```python
from build123d import *

# Parameters (mm, degrees)
CROQUIS1_W              = 45
CROQUIS1_H              = 45
SALIENTE_EXTRUIR1_DEPTH = 10
CORTAR_EXTRUIR1_DEPTH   = 10
CROQUIS3_W              = 26
CROQUIS3_H              = 26
CORTAR_EXTRUIR5_DEPTH   = 8
CROQUIS4_W              = 12
CROQUIS4_H              = 11
CORTAR_EXTRUIR6_DEPTH   = 4
CORTAR_EXTRUIR7_DEPTH   = 4
CROQUIS6_R              = 1.5
CORTAR_EXTRUIR8_DEPTH   = 24
CROQUIS7_R              = 1.5
CORTAR_EXTRUIR9_DEPTH   = 8


with BuildPart() as part:
    # Croquis1 → Saliente-Extruir1 (new body)
    with BuildSketch(Plane.XY):
        Rectangle(CROQUIS1_W, CROQUIS1_H)
    extrude(amount=SALIENTE_EXTRUIR1_DEPTH)

    # Croquis2 → Cortar-Extruir1 (cut)
    with BuildSketch(Plane.XY.offset(10)):
        with BuildLine():
            ThreePointArc((-11.5, -6), (-7.610912703, -7.610912703), (-6, -11.5))
            Line((-6, -11.5), (6, -11.5))
            ThreePointArc((6, -11.5), (7.610912703, -7.610912703), (11.5, -6))
            Line((11.5, -6), (11.5, 6))
            ThreePointArc((11.5, 6), (7.610912703, 7.610912703), (6, 11.5))
            Line((6, 11.5), (-6, 11.5))
            ThreePointArc((-6, 11.5), (-7.610912703, 7.610912703), (-11.5, 6))
            Line((-11.5, 6), (-11.5, -6))
        make_face()
    extrude(amount=-CORTAR_EXTRUIR1_DEPTH, mode=Mode.SUBTRACT)

    # Croquis3 → Cortar-Extruir5 (cut)
    with BuildSketch(Plane.XY.offset(10)):
        Rectangle(CROQUIS3_W, CROQUIS3_H)
    extrude(amount=-CORTAR_EXTRUIR5_DEPTH, mode=Mode.SUBTRACT)

    # Croquis4 → Cortar-Extruir6 (cut)
    with BuildSketch(Plane(origin=(0, 0, 0), x_dir=(-1, 0, 0), z_dir=(0, 0, -1))):
        with Locations((0, 17)):
            Rectangle(CROQUIS4_W, CROQUIS4_H)
    extrude(amount=-CORTAR_EXTRUIR6_DEPTH, mode=Mode.SUBTRACT)

    # Croquis5 → Cortar-Extruir7 (cut)
    with BuildSketch(Plane(origin=(0, 0, 0), x_dir=(-1, 0, 0), z_dir=(0, 0, -1))):
        with BuildLine():
            ThreePointArc((-7.6, 9), (-9.989949494, 9.989949494), (-9, 7.6))
            Line((-9, 7.6), (-9, 9))
            Line((-9, 9), (-7.6, 9))
        make_face()
        with BuildLine():
            Line((-9, 9), (-9, 7.6))
            ThreePointArc((-9, 7.6), (-8.010050506, 8.010050506), (-7.6, 9))
            Line((-7.6, 9), (-9, 9))
        make_face()
        with BuildLine():
            ThreePointArc((7.6, 9), (8.010050506, 8.010050506), (9, 7.6))
            Line((9, 7.6), (9, 9))
            Line((9, 9), (7.6, 9))
        make_face()
        with BuildLine():
            Line((9, 9), (9, 7.6))
            ThreePointArc((9, 7.6), (9.989949494, 8.010050506), (10.4, 9))
            ThreePointArc((10.4, 9), (9, 10.4), (7.6, 9))
            Line((7.6, 9), (9, 9))
        make_face()
        with BuildLine():
            ThreePointArc((9, -7.6), (8.010050506, -8.010050506), (7.6, -9))
            Line((7.6, -9), (9, -9))
            Line((9, -9), (9, -7.6))
        make_face()
        with BuildLine():
            Line((9, -9), (7.6, -9))
            ThreePointArc((7.6, -9), (9, -10.4), (10.4, -9))
            ThreePointArc((10.4, -9), (9.989949494, -8.010050506), (9, -7.6))
            Line((9, -7.6), (9, -9))
        make_face()
        with BuildLine():
            Line((-9, -7.6), (-9, -9))
            Line((-9, -9), (-7.6, -9))
            ThreePointArc((-7.6, -9), (-8.010050506, -8.010050506), (-9, -7.6))
        make_face()
        with BuildLine():
            Line((-7.6, -9), (-9, -9))
            Line((-9, -9), (-9, -7.6))
            ThreePointArc((-9, -7.6), (-9.989949494, -9.989949494), (-7.6, -9))
        make_face()
    extrude(amount=-CORTAR_EXTRUIR7_DEPTH, mode=Mode.SUBTRACT)

    # Croquis6 → Cortar-Extruir8 (cut)
    with BuildSketch(Plane(origin=(0, 0, 0), x_dir=(-1, 0, 0), z_dir=(0, 0, -1))):
        with Locations((-17.5, 17.5)):
            Circle(CROQUIS6_R)
        with Locations((-17.5, -17.5)):
            Circle(CROQUIS6_R)
        with Locations((17.5, -17.5)):
            Circle(CROQUIS6_R)
        with Locations((17.5, 17.5)):
            Circle(CROQUIS6_R)
    extrude(amount=-CORTAR_EXTRUIR8_DEPTH, mode=Mode.SUBTRACT)

    # Croquis7 → Cortar-Extruir9 (cut)
    # profile 1 of 4: a face of its own
    with BuildSketch(Plane(origin=(0, 0, 0), x_dir=(-1, 0, 0), z_dir=(0, 0, -1))):
        with BuildLine():
            Line((-22.5, 22.5), (-22.5, 10.5))
            ThreePointArc((-22.5, 10.5), (-14.014718626, 14.014718626), (-10.5, 22.5))
            Line((-10.5, 22.5), (-22.5, 22.5))
        make_face()
        with Locations((-17.5, 17.5)):
            Circle(CROQUIS7_R, mode=Mode.SUBTRACT)
    # profile 2 of 4: a face of its own
    with BuildSketch(Plane(origin=(0, 0, 0), x_dir=(-1, 0, 0), z_dir=(0, 0, -1))):
        with BuildLine():
            ThreePointArc((10.5, 22.5), (14.014718626, 14.014718626), (22.5, 10.5))
            Line((22.5, 10.5), (22.5, 22.5))
            Line((22.5, 22.5), (10.5, 22.5))
        make_face()
        with Locations((17.5, 17.5)):
            Circle(CROQUIS7_R, mode=Mode.SUBTRACT)
    # profile 3 of 4: a face of its own
    with BuildSketch(Plane(origin=(0, 0, 0), x_dir=(-1, 0, 0), z_dir=(0, 0, -1))):
        with BuildLine():
            Line((10.5, -22.5), (22.5, -22.5))
            Line((22.5, -22.5), (22.5, -10.5))
            ThreePointArc((22.5, -10.5), (14.014718626, -14.014718626), (10.5, -22.5))
        make_face()
        with Locations((17.5, -17.5)):
            Circle(CROQUIS7_R, mode=Mode.SUBTRACT)
    # profile 4 of 4: a face of its own
    with BuildSketch(Plane(origin=(0, 0, 0), x_dir=(-1, 0, 0), z_dir=(0, 0, -1))):
        with BuildLine():
            Line((-22.5, -22.5), (-10.5, -22.5))
            ThreePointArc((-10.5, -22.5), (-14.014718626, -14.014718626), (-22.5, -10.5))
            Line((-22.5, -10.5), (-22.5, -22.5))
        make_face()
        with Locations((-17.5, -17.5)):
            Circle(CROQUIS7_R, mode=Mode.SUBTRACT)
    extrude(amount=-CORTAR_EXTRUIR9_DEPTH, mode=Mode.SUBTRACT)


solid = part.part
```
Geometry: final body of the model. Coordinates: model frame, mm. A direction names the side the tool comes from. Coordinates: 2 decimals unless noted, no trailing zeros. Order: outer loops, then holes, each group sorted by start corner. A loop starts at its lowest first (then second) coordinate and runs counter-clockwise, first axis right, second up. Notation, with made-up numbers: (87, 52) - (94, 52) arc R29 cw to (94, 79) - close; hole circle Ø3 at (-6, 39). An arc over 180 degrees is marked (long way). Write each question's results on one line, items separated by ' | '.
1) Section C-C, the plane y = 17.5. Return loops of the section in (x, z), plus the area to 3 significant figures.
Results list:
outline: (-22.5, 8) - (-19, 8) - (-19, 10) - (-22.5, 10) - close; (-16, 8) - (-11.59, 8) - (-11.59, 0) - (-6, 0) - (-6, 4) - (6, 4) - (6, 0) - (11.59, 0) - (11.59, 8) - (16, 8) - (16, 10) - (-16, 10) - close; (19, 8) - (22.5, 8) - (22.5, 10) - (19, 10) - close | area: 215 mm^2
2) Pin query (flat end, axial travel): pin 1 (13 mm diameter, centred on x = -15, y = -18, fed in from -Z); pin 2 (3 mm diameter, centred on y = 19, z = 1, fed in from -X); pin 3 (3 mm diameter, centred on x = -17.5, z = 1, fed in from -Y); pin 4 (3 mm diameter, centred on x = -13, z = 3.5, fed in from -Y). Return the tip coordinate at first contact, or that it passes through.
Results list:
pin 1: z = 0 | pin 2: x = -11.59 | pin 3: y = -12.41 | pin 4: y = -17.7
3) Line query: line 1 (Y direction, x = 17.5, z = 9); line 2 (Y direction, x = 9, z = 1.1); line 3 (X direction, y = 6, z = 7.5). Output: solid intervals per line, ascending. Write a range as from..to.
Results list:
line 1: -22.5..-19, -16..16, 19..22.5 | line 2: -22.5..-10.4, -7.6..-6.6, 6.6..7.6, 10.4..22.5 | line 3: -22.5..-13, 13..22.5
4) Section D-D, the plane x = 17.5. Return loops of the section in (y, z).
Results list:
outline: (-22.5, 8) - (-19, 8) - (-19, 10) - (-22.5, 10) - close; (-16, 8) - (-11.59, 8) - (-11.59, 0) - (11.59, 0) - (11.59, 8) - (16, 8) - (16, 10) - (-16, 10) - close; (19, 8) - (22.5, 8) - (22.5, 10) - (19, 10) - close
5) Section A-A, the plane x = 3. Return loops of the section in (y, z), plus the area to 3 significant figures.
Results list:
outline: (-22.5, 0) - (-11.5, 0) - (-11.5, 2) - (-13, 2) - (-13, 10) - (-22.5, 10) - close; (13, 4) - (22.5, 4) - (22.5, 10) - (13, 10) - close | area: 155 mm^2
6) Section B-B, the plane z = 6.25. Return loops of the section in (x, y), plus the area to 3 significant figures.
Results list:
outline: (-22.5, -10.5) arc R12 cw to (-10.5, -22.5) - (10.5, -22.5) arc R12 cw to (22.5, -10.5) - (22.5, 10.5) arc R12 cw to (10.5, 22.5) - (-10.5, 22.5) arc R12 cw to (-22.5, 10.5) - close; hole (-13, -13) - (13, -13) - (13, 13) - (-13, 13) - close | area: 897 mm^2
7) Pull-direction query (X, two-part tool) for faces 4 (the flat face through (22.5, 0, 6)), 5 (the flat face through (0, -22.5, 6)), 6 (the cylindrical face through (18.61, 18.51, 8.99)), 7 (the cylindrical face through (-14.11, -13.92, 3.94)); classes: pulls with the +X half, pulls with the -X half, needs draft (parallel to the pull), parting line crosses it, or undercut.
Results list:
face 4: pulls with the +X half | face 5: needs draft | face 6: undercut | face 7: pulls with the -X half
8) Set-up query: faces 1 (the flat face through (11.5, 0, 1)), 2 (the flat face through (-9.7, -7.6, 2)), 3 (the flat face through (0, 18, 4)). Return all of +Z, -Z, +X, -X, +Y, -Y with unobstructed straight access to the full face (end or side cutting, diameter ignored); none if empty.
Results list:
face 1: +Z, -Z | face 2: +Z | face 3: -Z, +Y
